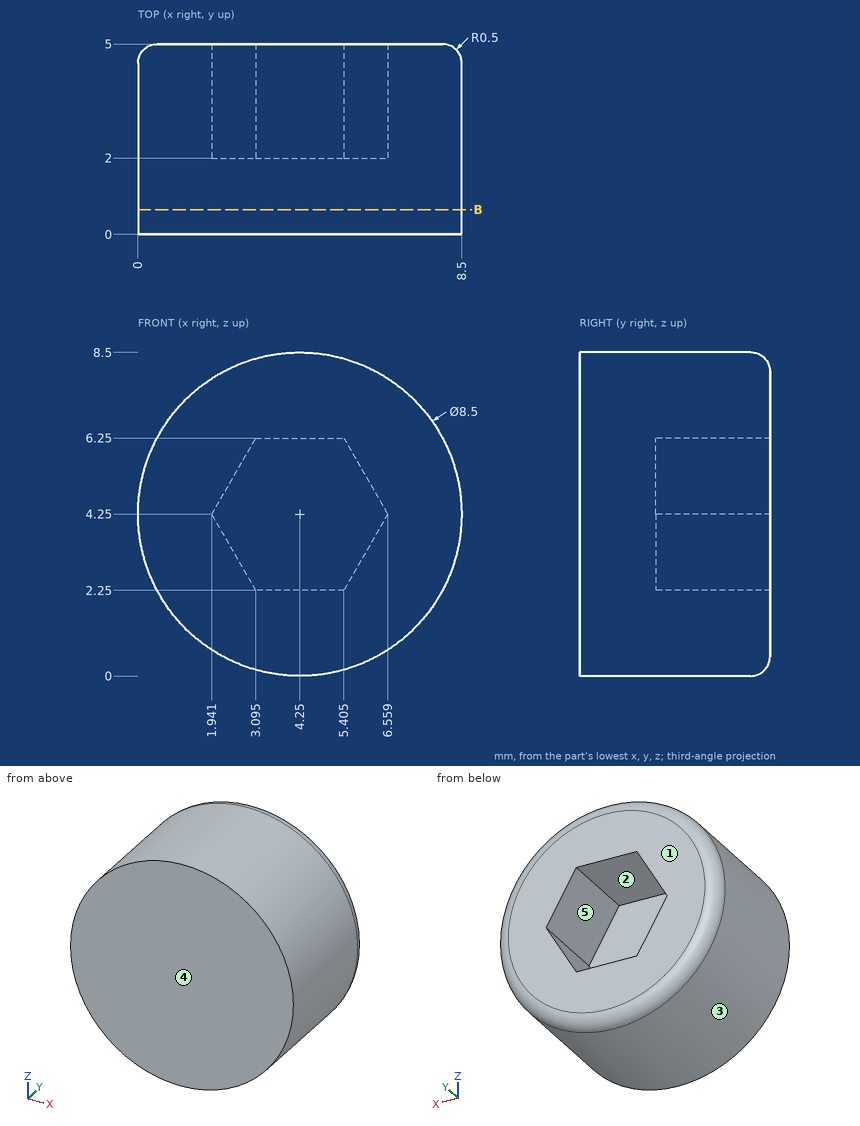
Input: dimensioned drawing with shaded views. Units: mm. Origin: part minimum x, y, z. A direction names the side the tool comes from. Give positions to 0.01 mm unless a question says otherwise; leave off trailing zeros. Order: outer loops, then holes, each group sorted by start corner. A loop starts at its lowest first (then second) coordinate and runs counter-clockwise, first axis right, second up. Notation, with made-up numbers: (79, 25.25) -> (90, 25.25) arc R14 ccw to (90, 39.25) -> close; hole circle Ø11 at (36.5, 89.5). An arc over 180 degrees is marked (long way). Answer as a JSON object with one key per item and string values.
Q1. Section B-B (y = 0.65). Output: boundary loops of the cut face in (x, z).
Entries:
{"outline": "circle Ø8.5 at (4.25, 4.25)"}
Q2. First-contact query: pin 1 (1.5 mm diameter, centred on y = 3.5, z = 2.5, fed in from -X); pin 2 (2 mm diameter, centred on x = 6, y = 3.5, fed in from +Z). Flat tips, straight axial feed; report the tip coordinate or a pass-through.
Entries:
{"pin 1": "stops at x = 0.12", "pin 2": "stops at z = 8.43"}
Q3. Draft query along X for the marked faces 1, 2 and 3. Return one class per face: released by +X, released by -X, zero draft, split by the parting line, or undercut.
Entries:
{"face 1": "zero draft", "face 2": "undercut", "face 3": "split by the parting line"}
Q4. Access query for the marked faces 4 and 5. Directions: +Z, -Z, +X, -X, +Y, -Y. A direction counts if a zero-diameter tool reaches every point of the face in a straight line with its end or side. Return the directions, or none.
Entries:
{"face 4": "+Z, -Z, +X, -X, -Y", "face 5": "+Y"}
Q5. Material intervals for probe 1 along Z at (x, y) = (4.25, 2.6); probe 2 along X at (y, z) = (2.65, 4) (1 decimal); probe 3 along Y at (x, z) = (3.25, 4), sorted ascending.
Entries:
{"probe 1": "z = 0 to 2.25, 6.25 to 8.5", "probe 2": "x = 0 to 2.1, 6.4 to 8.5", "probe 3": "y = 0 to 2"}
